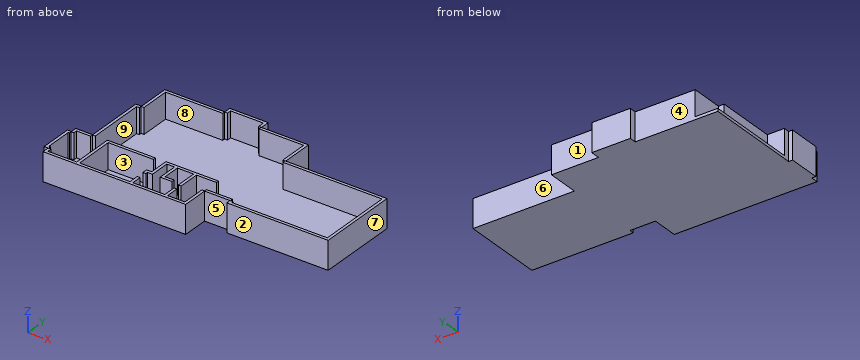
```python
from build123d import *

# Parameters (mm, degrees)
F0_W      = 6
F0_H      = 0.002
F0_W_2    = 1.4
F0_H_2    = 11.4
F0_W_3    = 13.6
F0_H_3    = 0.08
F0_H_4    = 16.002
F0_W_4    = 8.8
F0_H_5    = 21.098
F0_W_5    = 7.6
F0_H_6    = 7.8852218396
F1_DEPTH  = 1
F2_W      = 11.4
F2_H      = 9
F3_DEPTH  = 1
F4_W      = 1.4
F4_H      = 10
F5_DEPTH  = 1
F6_W      = 2.2483316878
F6_H      = 10
F7_DEPTH  = 1
F8_W      = 6
F8_H      = 10
F9_DEPTH  = 1
F10_W     = 21.2175605533
F10_H     = 10
F11_DEPTH = 1
F12_W     = 2
F12_H     = 10
F13_DEPTH = 1
F14_W     = 11.5231698511
F14_H     = 10
F15_DEPTH = 1
F16_W     = 21.2
F16_H     = 10
F17_DEPTH = 1
F18_W     = 2.4870870446
F18_H     = 10
F19_DEPTH = 1
F20_W     = 13.6
F20_H     = 10
F21_DEPTH = 1
F22_W     = 3.2888815676
F22_H     = 10
F23_DEPTH = 1
F24_W     = 16.7565354139
F24_H     = 9.9645610899
F25_DEPTH = 1
F26_W     = 11.2111184324
F26_H     = 9.9645610899
F27_DEPTH = 1
F28_W     = 35.9614706893
F28_H     = 10
F29_DEPTH = 1
F30_W     = 28.8
F30_H     = 10
F31_DEPTH = 1
F32_W     = 35.8
F32_H     = 10
F33_DEPTH = 1
F34_W     = 1.6
F34_H     = 10
F35_DEPTH = 1
F36_W     = 9.1939088942
F36_H     = 10
F37_DEPTH = 1
F38_W     = 9.3250730319
F38_H     = 10
F39_DEPTH = 1
F40_W     = 49.9146888159
F40_H     = 10
F41_DEPTH = 1
F42_W     = 50.4
F42_H     = 10
F43_DEPTH = 25.4
F44_W     = 2.4892
F44_H     = 10
F45_DEPTH = 1
F46_W     = 1.5276186168
F46_H     = 10
F47_DEPTH = 1
F48_W     = 8
F48_H     = 32.498
F49_DEPTH = 1
F50_W     = 1
F50_H     = 15
F50_H_2   = 1
F50_W_2   = 15.9833405107
F50_H_3   = 4.55
F50_H_4   = 2.7679902027
F50_H_5   = 0.7820097973
F50_H_6   = 6
F50_W_3   = 2.749538143
F50_H_7   = 7.5
F50_W_4   = 3.1995763704
F50_H_8   = 2.0981409718
F50_H_9   = 5.5018590282
F51_DEPTH = 9
F52_DEPTH = 9
F53_DEPTH = 9


with BuildPart() as f1:
    # F0 (on Top) → F1 (new body)
    with BuildSketch(Plane.XY):
        with Locations((-48.6298836529, -21.6088678897)):
            Rectangle(F0_W, F0_H)
        Polygon((-45.6298836529, -21.6098678897), (-51.6298836529, -21.6098678897), (-51.6298836529, -23.7206678897), (-51.6298836529, -35.1206678897), (-51.6298836529, -37.6098678897), (-40.4298836529, -37.6098678897), (-40.4298836529, -21.6098678897), align=None)
        Polygon((-45.6298836529, -21.6078678897), (-45.6298836529, -21.6098678897), (-40.4298836529, -21.6098678897), (-31.2298836529, -21.6098678897), (-31.2298836529, -21.6078678897), align=None)
        with Locations((-52.3298836529, -29.4206678897)):
            Rectangle(F0_W_2, F0_H_2)
        Polygon((-31.2298836529, -21.6098678897), (-40.4298836529, -21.6098678897), (-40.4298836529, -37.6098678897), (-22.4298836529, -37.6098678897), (-22.4298836529, -21.6078678897), (-31.2298836529, -21.6078678897), align=None)
        Polygon((-45.6298836529, -0.5098678897), (-45.6298836529, -21.6078678897), (-31.2298836529, -21.6078678897), (-31.2298836529, -0.5098678897), (-43.6298836529, -0.5098678897), align=None)
        with Locations((-15.6298836529, -37.6498678897)):
            Rectangle(F0_W_3, F0_H_3)
        with Locations((-15.6298836529, -29.6088678897)):
            Rectangle(F0_W_3, F0_H_4)
        Polygon((-43.6298836529, 10.8901321103), (-43.6298836529, -0.5098678897), (-31.2298836529, -0.5098678897), (-22.4298836529, -0.5098678897), (-22.4298836529, 10.8901321103), align=None)
        Polygon((-22.4298836529, -0.5098678897), (-22.4298836529, -21.6078678897), (-8.8298836529, -21.6078678897), (-8.8298836529, -13.7226460502), (-8.8298836529, 10.0012505427), (-8.8298836529, 13.2901321103), (-22.4298836529, 13.2901321103), (-22.4298836529, 10.8901321103), align=None)
        Polygon((-8.8298836529, -21.6078678897), (-8.8298836529, -37.6098678897), (-1.2298836529, -37.6098678897), (-1.2298836529, -28.4098678897), (-1.2298836529, -21.6078678897), align=None)
        Polygon((-8.8298836529, 10.0012505427), (-8.8298836529, -13.7226460502), (-1.2298836529, -13.7226460502), (7.7701163471, -13.7226460502), (7.7701163471, -1.2098678897), (7.7701163471, 10.0012505427), align=None)
        Polygon((-1.2298836529, -13.7226460502), (-1.2298836529, -21.6078678897), (-1.2298836529, -28.4098678897), (7.7701163471, -28.4098678897), (7.7701163471, -13.7226460502), align=None)
        Polygon((7.7701163471, -13.7226460502), (7.7701163471, -28.4098678897), (7.7701163471, -30.0098678897), (43.5701163471, -30.0098678897), (43.5701163471, -1.2098678897), (7.7701163471, -1.2098678897), align=None)
        with Locations((-26.8298836529, -11.0588678897)):
            Rectangle(F0_W_4, F0_H_5)
        with Locations((-5.0298836529, -17.6652569699)):
            Rectangle(F0_W_5, F0_H_6)
    extrude(amount=F1_DEPTH)

    # F2 (on face) → F3 (join)
    with BuildSketch(Plane(origin=(-53.0298836529, 0, 0), x_dir=(0, -1, 0), z_dir=(-1, 0, 0))):
        with Locations((29.4206678897, 5.5)):
            Rectangle(F2_W, F2_H)
    extrude(amount=-F3_DEPTH)

    # F4 (on face) → F5 (join)
    with BuildSketch(Plane(origin=(0, -23.7206678897, 0), x_dir=(-1, 0, 0), z_dir=(0, 1, 0))):
        with Locations((52.3298836529, 5)):
            Rectangle(F4_W, F4_H)
    extrude(amount=-F5_DEPTH)

    # F6 (on face) → F7 (join)
    with BuildSketch(Plane(origin=(-51.6298836529, 0, 0), x_dir=(0, -1, 0), z_dir=(-1, 0, 0))):
        with Locations((22.7320337336, 5)):
            Rectangle(F6_W, F6_H)
    extrude(amount=-F7_DEPTH)

    # F8 (on face) → F9 (join)
    with BuildSketch(Plane(origin=(0, -21.6078678897, 0), x_dir=(-1, 0, 0), z_dir=(0, 1, 0))):
        with Locations((48.6298836529, 5)):
            Rectangle(F8_W, F8_H)
    extrude(amount=-F9_DEPTH)

    # F10 (on face) → F11 (join)
    with BuildSketch(Plane(origin=(-45.6298836529, 0, 0), x_dir=(0, -1, 0), z_dir=(-1, 0, 0))):
        with Locations((11.1186481663, 5)):
            Rectangle(F10_W, F10_H)
    extrude(amount=-F11_DEPTH)

    # F12 (on face) → F13 (join)
    with BuildSketch(Plane(origin=(0, -0.5098678897, 0), x_dir=(-1, 0, 0), z_dir=(0, 1, 0))):
        with Locations((44.6298836529, 5)):
            Rectangle(F12_W, F12_H)
    extrude(amount=-F13_DEPTH)

    # F14 (on face) → F15 (join)
    with BuildSketch(Plane(origin=(-43.6298836529, 0, 0), x_dir=(0, -1, 0), z_dir=(-1, 0, 0))):
        with Locations((-5.1285471847, 5)):
            Rectangle(F14_W, F14_H)
    extrude(amount=-F15_DEPTH)

    # F16 (on face) → F17 (join)
    with BuildSketch(Plane(origin=(0, 10.8901321103, 0), x_dir=(-1, 0, 0), z_dir=(0, 1, 0))):
        with Locations((33.0298836529, 5)):
            Rectangle(F16_W, F16_H)
    extrude(amount=-F17_DEPTH)

    # F18 (on face) → F19 (join)
    with BuildSketch(Plane(origin=(-22.4298836529, 0, 0), x_dir=(0, -1, 0), z_dir=(-1, 0, 0))):
        with Locations((-12.046588588, 5)):
            Rectangle(F18_W, F18_H)
    extrude(amount=-F19_DEPTH)

    # F20 (on face) → F21 (join)
    with BuildSketch(Plane(origin=(0, 13.2901321103, 0), x_dir=(-1, 0, 0), z_dir=(0, 1, 0))):
        with Locations((15.6298836529, 5)):
            Rectangle(F20_W, F20_H)
    extrude(amount=-F21_DEPTH)

    # F22 (on face) → F23 (join)
    with BuildSketch(Plane.YZ.offset(-8.8298836529)):
        with Locations((11.6456913265, 5)):
            Rectangle(F22_W, F22_H)
    extrude(amount=-F23_DEPTH)

    # F24 (on face) → F25 (join)
    with BuildSketch(Plane(origin=(0, 10.0012505427, 0), x_dir=(-1, 0, 0), z_dir=(0, 1, 0))):
        with Locations((0.6081513599, 4.9822805449)):
            Rectangle(F24_W, F24_H)
    extrude(amount=-F25_DEPTH)

    # F26 (on face) → F27 (join)
    with BuildSketch(Plane.YZ.offset(7.7701163471)):
        with Locations((4.3956913265, 4.9822805449)):
            Rectangle(F26_W, F26_H)
    extrude(amount=-F27_DEPTH)

    # F28 (on face) → F29 (join)
    with BuildSketch(Plane(origin=(0, -1.2098678897, 0), x_dir=(-1, 0, 0), z_dir=(0, 1, 0))):
        with Locations((-25.5893810024, 5)):
            Rectangle(F28_W, F28_H)
    extrude(amount=-F29_DEPTH)

    # F30 (on face) → F31 (join)
    with BuildSketch(Plane.YZ.offset(43.5701163471)):
        with Locations((-15.6098678897, 5)):
            Rectangle(F30_W, F30_H)
    extrude(amount=-F31_DEPTH)

    # F32 (on face) → F33 (join)
    with BuildSketch(Plane.XZ.offset(30.0098678897)):
        with Locations((25.6701163471, 5)):
            Rectangle(F32_W, F32_H)
    extrude(amount=-F33_DEPTH)

    # F34 (on face) → F35 (join)
    with BuildSketch(Plane(origin=(7.7701163471, 0, 0), x_dir=(0, -1, 0), z_dir=(-1, 0, 0))):
        with Locations((29.2098678897, 5)):
            Rectangle(F34_W, F34_H)
    extrude(amount=-F35_DEPTH)

    # F36 (on face) → F37 (join)
    with BuildSketch(Plane.XZ.offset(28.4098678897)):
        with Locations((3.3670707942, 5)):
            Rectangle(F36_W, F36_H)
    extrude(amount=-F37_DEPTH)

    # F38 (on face) → F39 (join)
    with BuildSketch(Plane.YZ.offset(-1.2298836529)):
        with Locations((-32.9473313738, 5)):
            Rectangle(F38_W, F38_H)
    extrude(amount=-F39_DEPTH)

    # F40 (on face) → F41 (join)
    with BuildSketch(Plane.XZ.offset(37.6098678897)):
        with Locations((-26.672539245, 5)):
            Rectangle(F40_W, F40_H)
    extrude(amount=-F41_DEPTH)

    # F42 (on face) → F43 (cut)
    with BuildSketch(Plane.XZ.offset(37.6098678897)):
        with Locations((-26.4298836529, 5)):
            Rectangle(F42_W, F42_H)
    extrude(amount=F43_DEPTH, mode=Mode.SUBTRACT)

    # F44 (on face) → F45 (join)
    with BuildSketch(Plane(origin=(-51.6298836529, 0, 0), x_dir=(0, -1, 0), z_dir=(-1, 0, 0))):
        with Locations((36.3652678897, 5)):
            Rectangle(F44_W, F44_H)
    extrude(amount=-F45_DEPTH)

    # F46 (on face) → F47 (join)
    with BuildSketch(Plane.XZ.offset(35.1206678897)):
        with Locations((-52.2660743445, 5)):
            Rectangle(F46_W, F46_H)
    extrude(amount=-F47_DEPTH)

    # F48 (on Top) → F49 (join)
    with BuildSketch(Plane.XY):
        with Locations((-47.6298836529, -5.3588678897)):
            Rectangle(F48_W, F48_H)
    extrude(amount=F49_DEPTH)

    # F50 (on face) → F51 (join)
    with BuildSketch(Plane.XY.offset(1)):
        with Locations((-39.9298836529, -30.1098678897)):
            Rectangle(F50_W, F50_H)
        with Locations((-39.9298836529, -22.1098678897)):
            Rectangle(F50_W, F50_H_2)
        with Locations((-31.4382133976, -22.1098678897)):
            Rectangle(F50_W_2, F50_H_2)
        with Locations((-21.1280035675, -35.3348678897)):
            Rectangle(F50_W, F50_H_3)
        with Locations((-21.1280035675, -31.6758727883)):
            Rectangle(F50_W, F50_H_4)
        with Locations((-21.1280035675, -29.9008727883)):
            Rectangle(F50_W, F50_H_5)
        with Locations((-21.1280035675, -29.0098678897)):
            Rectangle(F50_W, F50_H_2)
        Polygon((-20.6280035675, -28.5098678897), (-20.6280035675, -29.5098678897), (-18.8280035675, -29.5098678897), (-18.8280035675, -28.5098678897), (-19.8280035675, -28.5098678897), align=None)
        with Locations((-19.3280035675, -25.5098678897)):
            Rectangle(F50_W, F50_H_6)
        with Locations((-19.3280035675, -22.0098678897)):
            Rectangle(F50_W, F50_H_2)
        with Locations((-17.4532344959, -22.0098678897)):
            Rectangle(F50_W_3, F50_H_2)
        with Locations((-15.5784654244, -22.0098678897)):
            Rectangle(F50_W, F50_H_2)
        with Locations((-15.5784654244, -25.5098678897)):
            Rectangle(F50_W, F50_H_6)
        Polygon((-15.0784654244, -21.5098678897), (-15.0784654244, -22.5098678897), (-9.3298836529, -22.5098678897), (-9.3298836529, -22.4098678897), (-8.3298836529, -22.4098678897), (-8.3298836529, -21.5098678897), align=None)
        with Locations((-15.5784654244, -29.0098678897)):
            Rectangle(F50_W, F50_H_2)
        with Locations((-8.8298836529, -26.2598678897)):
            Rectangle(F50_W, F50_H_7)
        Polygon((-9.3298836529, -22.4098678897), (-9.3298836529, -22.5098678897), (-8.3298836529, -22.5098678897), (-8.3298836529, -22.5030053407), (-8.3298836529, -22.4098678897), align=None)
        with Locations((-13.4786772393, -29.0098678897)):
            Rectangle(F50_W_4, F50_H_2)
        Polygon((-1.3298836529, -21.5098678897), (-8.3298836529, -21.5098678897), (-8.3298836529, -22.4098678897), (-8.3298836529, -22.5030053407), (-1.3298836529, -22.5030053407), align=None)
        with Locations((-8.8298836529, -31.0589383756)):
            Rectangle(F50_W, F50_H_8)
        with Locations((-8.8298836529, -34.8589383756)):
            Rectangle(F50_W, F50_H_9)
    extrude(amount=F51_DEPTH)

    # F50 (on face) → F52 (cut)
    with BuildSketch(Plane.XY.offset(1)):
        with Locations((-21.1280035675, -31.6758727883)):
            Rectangle(F50_W, F50_H_4)
    extrude(amount=F52_DEPTH, mode=Mode.SUBTRACT)

    # F50 (on face) → F53 (cut)
    with BuildSketch(Plane.XY.offset(1)):
        with Locations((-8.8298836529, -31.0589383756)):
            Rectangle(F50_W, F50_H_8)
    extrude(amount=F53_DEPTH, mode=Mode.SUBTRACT)


solid = f1.part
```
Design review of the part built by this model. Coordinates are the model's own, in mm. Face numbers are marked on the shaded views. A direction names the side the tool comes from. Coordinates: 2 decimals unless noted, no trailing zeros. Loops run counter-clockwise (first coordinate to the right, second up) from the corner with the lowest first, then second, coordinate; pieces in that order, holes last. Notation, with made-up numbers: (-25, 6.25) -> (5, 6.25) arc R4 ccw to (5, 13.25) -> close; hole circle Ø11 at (-16.75, 23). An arc over 180 degrees is marked (long way). Answer as a JSON object with one key per item and string values.
Q1. The part is to be moulded in two halves that separate along Y. For the marked faces 6, 7, 8 and 9, say which applies: +Y half, -Y half, draft (parallel to the pull), parting line (faces both ways), or undercut.
Answer block:
{"face 6": "+Y half", "face 7": "draft", "face 8": "undercut", "face 9": "undercut"}
Q2. Take a section at D-D on y = -8.5. Give the boundary of the cut face in (x, z).
Answer block:
{"outline": "(-51.63, 0) -> (43.57, 0) -> (43.57, 10) -> (42.57, 10) -> (42.57, 1) -> (-44.63, 1) -> (-44.63, 10) -> (-45.63, 10) -> (-45.63, 1) -> (-51.63, 1) -> close"}
Q3. Take a section at C-C on x = 35. Give the boundary of the cut face in (y, z).
Answer block:
{"outline": "(-30.01, 0) -> (-1.21, 0) -> (-1.21, 10) -> (-2.21, 10) -> (-2.21, 1) -> (-29.01, 1) -> (-29.01, 10) -> (-30.01, 10) -> close"}
Q4. To check wall thickness, follow L1, parallel to X at y = -34.5, z = 3; L2, parallel to Y at x = -23.5, z = 8; L3, parallel to X at y = -23.5, z = 2.5. State the ranges of each line that lie inside material, in increasing order.
Answer block:
{"L1": "x = -53.03 to -51.5, -40.43 to -39.43, -21.63 to -20.63, -9.33 to -8.33, -2.23 to -1.23", "L2": "y = -37.61 to -36.61, -22.61 to -21.61, 9.89 to 10.89", "L3": "x = -51.63 to -50.63, -40.43 to -39.43, -19.83 to -18.83, -16.08 to -15.08, -9.33 to -8.33, 42.57 to 43.57"}
Q5. Tool access review of the marked faces 1, 2, 3, 4 and 5: name each direction out of +Z, -Z, +X, -X, +Y, -Y from which nothing blocks a thin tool from reaching the whole face with its end or side.
Answer block:
{"face 1": "+Z, -Z, +X, +Y", "face 2": "+Z, -Z, +X, -Y", "face 3": "+Z", "face 4": "+Z, -Z, -X, +Y", "face 5": "+Z, -Z, -Y"}
Q6. Take a section at B-B on z = 2.75. Give the number of separate pieces and of enclosed holes in the cut face, plus the area to 3 significant figures.
Answer block:
{"separate pieces": "2", "enclosed holes": "1", "area": "371 mm^2"}
Q7. Take a section at A-A on y = 8. Give the boundary of the cut face in (x, z), plus the area to 3 significant figures.
Answer block:
{"outline": "(-51.63, 0) -> (7.77, 0) -> (7.77, 9.96) -> (6.77, 9.96) -> (6.77, 1) -> (-42.63, 1) -> (-42.63, 10) -> (-43.63, 10) -> (-43.63, 1) -> (-51.63, 1) -> close", "area": "77.4 mm^2"}
Q8. Clearance check with flat-ended pins moving along their axes: pin 1 Ø10 at (x, y) = (-9.5, -4.5) entering from +Z; pin 2 Ø5 at (x, z) = (-40.5, 7) entering from +Y; pin 3 Ø2 at (x, y) = (25.5, -22) entering from -Z; pin 4 Ø2.5 at (x, z) = (2, 3.5) entering from -Y. State where each tip first meets the part, or that it passes through.
Answer block:
{"pin 1": "stops at z = 1", "pin 2": "stops at y = 10.89", "pin 3": "stops at z = 0", "pin 4": "stops at y = -28.41"}
